from build123d import *

# Parameters (mm, degrees)
SKETCH1_R             = 3.175
BOSS_EXTRUDE1_DEPTH   = 4.7625
BOSS_EXTRUDE1_2_DEPTH = 4.7625
BOSS_EXTRUDE1_3_DEPTH = 4.7625
BOSS_EXTRUDE1_4_DEPTH = 4.7625
BOSS_EXTRUDE1_5_DEPTH = 4.7625
SKETCH2_R             = 1.984375
BOSS_EXTRUDE2_DEPTH   = 9.525
BOSS_EXTRUDE3_DEPTH   = 3.175
CHAMFER1_SIZE         = 9.081162376
CHAMFER1_SIZE_2       = 7.62


with BuildPart() as part:
    # Sketch1 → Boss-Extrude1 (new body)
    with BuildSketch(Plane.XY):
        with Locations(Location((-78.19292114, 62.356773808, 0), (0, 0, 180))):
            Circle(SKETCH1_R)
    extrude(amount=BOSS_EXTRUDE1_DEPTH)



with BuildPart() as body_2:
    # Sketch1 → Boss-Extrude1 2 (new body)
    with BuildSketch(Plane.XY):
        with Locations(Location((-97.504977817, -22.254874907, 0), (0, 0, 180))):
            Circle(SKETCH1_R)
    extrude(amount=BOSS_EXTRUDE1_2_DEPTH)


with BuildPart() as body_3:
    # Sketch1 → Boss-Extrude1 3 (new body)
    with BuildSketch(Plane.XY):
        with Locations(Location((-43.393797458, -90.108148901, 0), (0, 0, 180))):
            Circle(SKETCH1_R)
    extrude(amount=BOSS_EXTRUDE1_3_DEPTH)


with BuildPart() as body_4:
    # Sketch1 → Boss-Extrude1 4 (new body)
    with BuildSketch(Plane.XY):
        with BuildLine():
            Line((-88.191845565, 53.571060584), (-82.764655069, 50.274379933))
            ThreePointArc((-82.764655069, 50.274379933), (-94.409581696, 21.548370942), (-96.381613527, -9.385413164))
            Line((-96.381613527, -9.385413164), (-102.701719332, -10.000850093))
            ThreePointArc((-102.701719332, -10.000850093), (-100.600373938, 22.961378873), (-88.191845565, 53.571060584))
        make_face()
    extrude(amount=BOSS_EXTRUDE1_4_DEPTH)


with BuildPart() as body_5:
    # Sketch1 → Boss-Extrude1 5 (new body)
    with BuildSketch(Plane.XY):
        with BuildLine():
            Line((-90.909011383, -33.362449786), (-96.870258031, -35.550151411))
            ThreePointArc((-96.870258031, -35.550151411), (-80.675236097, -64.336353929), (-56.214495182, -86.53086552))
            Line((-56.214495182, -86.53086552), (-52.755141633, -81.20588918))
            ThreePointArc((-52.755141633, -81.20588918), (-75.710606183, -60.377193687), (-90.909011383, -33.362449786))
        make_face()
    extrude(amount=BOSS_EXTRUDE1_5_DEPTH)


with BuildPart() as part_1:
    add(part.part)

    add(body_2.part)  # Boss-Extrude2 merges body 2

    add(body_3.part)  # Boss-Extrude2 merges body 3
    # Sketch2 → Boss-Extrude2 (add)
    with BuildSketch(Plane.XY):
        with BuildLine():
            Line((-82.430084054, 80.927094637), (-136.637001873, 66.402394783))
            ThreePointArc((-136.637001873, 66.402394783), (-143.425587422, 61.866406938), (-146.05, 54.13513679))
            Line((-146.05, 54.13513679), (-146.05, -127))
            ThreePointArc((-146.05, -127), (-140.470384182, -140.470384182), (-127, -146.05))
            Line((-127, -146.05), (-51.469574148, -146.05))
            ThreePointArc((-51.469574148, -146.05), (-43.738303999, -143.425587422), (-39.202316154, -136.637001873))
            Line((-39.202316154, -136.637001873), (-29.247808511, -99.486273586))
            ThreePointArc((-29.247808511, -99.486273586), (-30.083781104, -90.666124862), (-36.482937232, -84.53875393))
            ThreePointArc((-36.482937232, -84.53875393), (-89.766487514, -20.488614994), (-69.549981311, 60.337432202))
            ThreePointArc((-69.549981311, 60.337432202), (-68.376222335, 75.395171012), (-82.430084054, 80.927094637))
        make_face()
        with Locations((-136.525, 44.45)):
            Circle(SKETCH2_R, mode=Mode.SUBTRACT)
        with Locations((-136.525, -31.75)):
            Circle(SKETCH2_R, mode=Mode.SUBTRACT)
        with Locations((-136.525, -107.95)):
            Circle(SKETCH2_R, mode=Mode.SUBTRACT)
        with Locations((-57.15, -136.525)):
            Circle(SKETCH2_R, mode=Mode.SUBTRACT)
        with Locations((-107.95, -136.525)):
            Circle(SKETCH2_R, mode=Mode.SUBTRACT)
    extrude(amount=-BOSS_EXTRUDE2_DEPTH)


    add(body_4.part)  # Boss-Extrude3 merges body 4

    add(body_5.part)  # Boss-Extrude3 merges body 5
    # Sketch3 → Boss-Extrude3 (add)
    with BuildSketch(Plane.XY.offset(4.7625)):
        with BuildLine():
            Line((-81.407857445, 49.45020977), (-88.191845565, 53.571060584))
            ThreePointArc((-88.191845565, 53.571060584), (-100.600373938, 22.961378873), (-102.701719332, -10.000850093))
            Line((-102.701719332, -10.000850093), (-94.801587075, -9.231553932))
            ThreePointArc((-94.801587075, -9.231553932), (-92.861883635, 21.195118959), (-81.407857445, 49.45020977))
        make_face()
        with BuildLine():
            Line((-96.870258031, -35.550151411), (-89.418699721, -32.815524379))
            ThreePointArc((-89.418699721, -32.815524379), (-74.469448705, -59.387403627), (-51.890303245, -79.874645095))
            Line((-51.890303245, -79.874645095), (-56.214495182, -86.53086552))
            ThreePointArc((-56.214495182, -86.53086552), (-80.675236097, -64.336353929), (-96.870258031, -35.550151411))
        make_face()
    extrude(amount=-BOSS_EXTRUDE3_DEPTH)

    # Chamfer1
    # the kernel refuses this chamfer: 9.081162376, 7.62 mm, written as the material it takes off along each edge
    with BuildSketch(Plane(origin=(0, 0, -9.525), x_dir=(-0.15246082974719, -0.9883095139645264, 0), z_dir=(0.9883095139645264, -0.15246082974719, 0))) as chamfer1_piece_1:
        Polygon((92.075 + CHAMFER1_SIZE, 0), (92.075, -CHAMFER1_SIZE_2), (92.075, 0), align=None)
    revolve(axis=Axis((0, 0, -9.525), (0, 0, -1)), revolution_arc=136.746589735, mode=Mode.SUBTRACT)


solid = part_1.part
Design review of the part built by this model. Coordinates are the model's own, in mm. A direction names the side the tool comes from. Coordinates: 2 decimals unless noted, no trailing zeros. Order: outer loops, then holes, each group sorted by start corner. A loop starts at its lowest first (then second) coordinate and runs counter-clockwise, first axis right, second up.
Item 1: Take a section at A-A, the plane z = -5.5. Write out the cut boundary in (x, y) (3 decimals), then the cut area to 3 significant figures.
Item 2: Take a section at C-C, the plane y = -123. Write out the cut boundary in (x, z) (3 decimals).
Item 3: For faces 5 (the cylindrical face through (-75.438, -60.717, 0.783)), 6 (the cylindrical face through (-92.956, 20.777, 3.197)), 7 (the cylindrical face through (-80.964, -63.973, 2.348)), 8 (the cylindrical face through (-40.87, -88.18, 2.35)), list the 3-axis set-ups (+Z, -Z, +X, -X, +Y, -Y) from which the entire face can be reached by the end or side of a thin tool; tool diameter is ignored.
Item 4: For line 1 (Z direction, x = -109.5, y = -39.5) (3 decimals); line 2 (Y direction, x = -108, z = -5.25); line 3 (Y direction, x = -95, z = -1.25), list the stretches that pass through material, from the lowest coordinate up.
Item 5: For pin 1 Ø8 at (x, y) = (-112, -61.5) entering from +Z; pin 2 Ø8 at (y, z) = (-45.5, 0.5) entering from +X; pin 3 Ø3 at (x, y) = (-136.525, -31.75) entering from +Z; pin 4 Ø1.5 at (x, z) = (-134, -3.5) entering from +Y, all flat-tipped, find the tip position at first contact; note any pin that passes through.
Item 6: The part is to be moulded in two halves that separate along Y. For faces 1 (the cylindrical face through (-94.312, 21.973, 0.783)), 2 (the flat face through (-90, -146.05, -5)), 3 (the flat face through (-101, -56, -9.525)), 4 (the cylindrical face through (-136.955, 42.513, -4.696)), say which applies: pulls with the +Y half, pulls with the -Y half, needs draft (parallel to the pull), parting line crosses it, or undercut.
The answers:
1. outline: (-146.05, -127) arc R19.05 ccw to (-127, -146.05) - (-51.47, -146.05) arc R12.7 ccw to (-39.202, -136.637) - (-29.248, -99.486) arc R12.7 ccw to (-29.644, -91.686) arc R96.359 cw to (-66.489, 69.744) arc R12.7 ccw to (-82.43, 80.927) - (-136.637, 66.402) arc R12.7 ccw to (-146.05, 54.135) - close; hole circle Ø3.969 at (-136.525, -107.95); hole circle Ø3.969 at (-136.525, -31.75); hole circle Ø3.969 at (-136.525, 44.45); hole circle Ø3.969 at (-107.95, -136.525); hole circle Ø3.969 at (-57.15, -136.525)
1. area: 16,500 mm2
2. outline: (-146.05, -9.525) - (-35.548, -9.525) - (-35.548, 0) - (-146.05, 0) - close
3. face 5: +X
3. face 6: +Z, +X
3. face 7: +Z, -X, -Y
3. face 8: +Z
4. line 1: z = -9.525 to 0
4. line 2: y = -146.05 to -138.51, -134.54 to 74.08
4. line 3: y = -146.05 to 77.56
5. pin 1: stops at z = 0
5. pin 2: stops at x = -77.66
5. pin 3: passes through
5. pin 4: stops at y = 67.31
6. face 1: undercut
6. face 2: pulls with the -Y half
6. face 3: needs draft
6. face 4: undercut
